For this review, take the finished solid that the model builds, in its own axes (mm). A direction names the side the tool comes from. Coordinates: 2 decimals unless noted, no trailing zeros. Order: outer loops, then holes, each group sorted by start corner. A loop starts at its lowest first (then second) coordinate and runs counter-clockwise, first axis right, second up.
from build123d import *

# Parameters (mm, degrees)
F0_W     = 124
F0_H     = 228
F1_DEPTH = 15
F2_W     = 124
F2_H     = 203
F3_DEPTH = 35
F5_W     = 10
F5_H     = 15
F6_DEPTH = 2
F7_D     = 4.4


with BuildPart() as f1:
    # F0 (on Top) → F1 (new body)
    with BuildSketch(Plane.XY):
        Rectangle(F0_W, F0_H)
    extrude(amount=F1_DEPTH)

    # F2 (on face) → F3 (join)
    with BuildSketch(Plane.XY.offset(15)):
        with Locations((0, 12.5)):
            Rectangle(F2_W, F2_H)
    extrude(amount=F3_DEPTH)

    # F5 (on face) → F6 (join)
    with BuildSketch(Plane(origin=(0, 0, 0), x_dir=(1, 0, 0), z_dir=(0, 0, -1))):
        with Locations((-57, 121.5)):
            Rectangle(F5_W, F5_H)
        with Locations((57, 121.5)):
            Rectangle(F5_W, F5_H)
        with Locations((57, -121.5)):
            Rectangle(F5_W, F5_H)
        with Locations((-57, -121.5)):
            Rectangle(F5_W, F5_H)
    extrude(amount=-F6_DEPTH)

    # F7 (through all)
    with Locations(Plane(origin=(0, 0, 0), x_dir=(1, 0, 0), z_dir=(0, 0, -1))):
        with Locations((57.5, -121), (-57.5, -121), (-57.5, 121), (57.5, 121)):
            Hole(F7_D / 2)


solid = f1.part
1. Take a section at B-B, the plane z = 40.5. Give the boundary of the cut face in (x, y), plus the area to 3 significant figures.
Answer below:
outline: (-62, -89) - (62, -89) - (62, 114) - (-62, 114) - close
area: 25,200 mm2
2. The part is to be moulded in two halves that separate along X. For faces 4 (the face through (-1, -2, 0)), 5 (the face through (-58.683, 119.145, 1.014)), 6 (the face through (-62, 2, 25)), say which applies: +X half, -X half, draft (parallel to the pull), parting line (faces both ways), or undercut.
Answer below:
face 4: draft
face 5: undercut
face 6: -X half
3. Take a section at A-A, the plane x = 20. Give the boundary of the cut face in (y, z).
Answer below:
outline: (-114, 0) - (114, 0) - (114, 50) - (-89, 50) - (-89, 15) - (-114, 15) - close
4. Clearance check with flat-ended pins moving along their axes: pin 1 Ø5 at (x, y) = (56, 120) entering from +Z; pin 2 Ø4.5 at (x, z) = (9, 9) entering from -Y; pin 3 Ø8 at (x, z) = (-30, 14) entering from +Y; pin 4 Ø2.5 at (x, y) = (-57.5, -121) entering from -Z. State where each tip first meets the part, or that it passes through.
Answer below:
pin 1: stops at z = 2
pin 2: stops at y = -114
pin 3: stops at y = 114
pin 4: passes through
5. To check wall thickness, follow L1, parallel to X at y = 121, z = 1; L2, parallel to Y at x = 57.5, z = 0.4; L3, parallel to Y at x = -33.5, z = 25. State the ranges of each line that lie inside material, in increasing order.
Answer below:
L1: x = -62 to -59.7, -55.3 to -52, 52 to 55.3, 59.7 to 62
L2: y = -129 to -123.2, -118.8 to 118.8, 123.2 to 129
L3: y = -89 to 114
6. Machinability: for faces 1 (the face through (56.9, -123.3, 2)), 2 (the face through (56.317, 119.145, 1.014)), 3 (the face through (-56, 123, 2)), which of the approach directions +Z, -Z, +X, -X, +Y, -Y give a long, thin tool a straight path to every point of the face, cutting with its end or side? Answer none if there is none.
Answer below:
face 1: +Z, +X, -X, -Y
face 2: +Z, -Z
face 3: +Z, +X, -X, +Y
7. Take a section at C-C, the plane y = -98.5. Give the boundary of the cut face in (x, z).
Answer below:
outline: (-62, 0) - (62, 0) - (62, 15) - (-62, 15) - close
